Verification items for the finished model (mm, model axes). A direction names the side the tool comes from. Round coordinates to 2 decimals unless told otherwise and drop trailing zeros. Loops run counter-clockwise (first coordinate to the right, second up) from the corner with the lowest first, then second, coordinate; pieces in that order, holes last. Notation, with made-up numbers: M -33,83.25 L -27,83.25 A16 cw -27,99.25 Z; hole C -29,-7 d1. An arc over 180 degrees is marked long. One line per item, written item: value.
Autodesk Inventor part; units mm, degrees
ref_plane "YZ Plane" through (0, 0, 0) normal (1, 0, 0) x (0, 1, 0)
ref_plane "XZ Plane" through (0, 0, 0) normal (0, 1, 0) x (-1, 0, 0)
ref_plane "XY Plane" through (0, 0, 0) normal (0, 0, 1) x (1, 0, 0)
sketch "Sketch1" plane through (0, 0, 0) normal (0, 0, 1) x (1, 0, 0)
  circle A0 centre (0, 0) radius 1.75
  arc A1 (-16.5, -1.75) -> (-16.5, 1.75) centre (-16.5, 0) ccw
  arc A2 (-17.5, 1.75) -> (-17.5, -1.75) centre (-17.5, 0) ccw
  line L0 (-17.5, 1.75) -> (-16.5, 1.75)
  line L1 (-17.5, -1.75) -> (-16.5, -1.75)
  arc A3 (15.9971, -4.4051) -> (14.7172, -7.6627) centre (15.3572, -6.0339) ccw
  arc A4 (15.6479, -8.0283) -> (16.9279, -4.7708) centre (16.2879, -6.3996) ccw
  line L2 (15.6479, -8.0283) -> (14.7172, -7.6627)
  line L3 (16.9279, -4.7708) -> (15.9971, -4.4051)
  circle A5 centre (16.2879, -6.3996) radius 3
  circle A6 centre (-17.5, 0) radius 3
  circle A7 centre (0, 0) radius 2.25
  line L4 (-17.3714, 2.9972) -> (0.0964, 2.2479)
  line L5 (17.2643, -3.5629) -> (0.7323, 2.1275)
  line L6 (-17.6714, -2.9951) -> (-2.0561, -3.8889)
  line L7 (15.3522, -9.2499) -> (0.4916, -4.3714)
  arc A8 (0.4916, -4.3714) -> (-2.0561, -3.8889) centre (-2.6275, -13.8725) ccw
  circle A9 centre (-2.5071, -13.2368) radius 3.25
  circle A10 centre (-2.5071, -13.2368) radius 6
  line L8 (-19.8004, -1.9257) -> (-7.1079, -17.0881)
  line L9 (17.7248, -9.0331) -> (0.3666, -18.5038)
  dimension "d0" = 3.5
  dimension "d1" = 3.5
  dimension "d2" = 3.5
  dimension "d5" = 158.55
  dimension "d7" = 6
  dimension "d9" = 6
  dimension "d10" = 4.5
  dimension "d11" = 10
  dimension "d14" = 0
  dimension "d15" = 0
  dimension "d18" = 6.5
  dimension "d19" = 12
  dimension "d20" = 20
  dimension "d21" = 20
extrude "Extrusion1" add sketch "Sketch1" along normal blind 5
properties part number "CoinLockOpener"
(1) Sectioned sample at C-C on y = 0. Enter the section's corners in (x, z), and give its area (3 significant figures).
Completed:
outline: M -20.5,0 L -19.25,0 L -19.25,5 L -20.5,5 Z; M -14.75,0 L -1.75,0 L -1.75,5 L -14.75,5 Z; M 1.75,0 L 6.91,0 L 6.91,5 L 1.75,5 Z
area: 97.1 mm^2
(2) Sectioned sample at A-A on y = -6. Enter the section's corners in (x, z), and give its area (3 significant figures).
Completed:
outline: M -16.39,0 L 13.61,0 L 13.61,5 L -16.39,5 Z; M 17.99,0 L 19.26,0 L 19.26,5 L 17.99,5 Z
area: 156 mm^2
(3) Sectioned sample at B-B on x = -5. Enter the section's corners in (y, z).
Completed:
outline: M -18.69,0 L -15.32,0 L -15.32,5 L -18.69,5 Z; M -11.15,0 L 2.47,0 L 2.47,5 L -11.15,5 Z
(4) Tool access check on faces 1 (the face through (-8.76, 2.628, 2.465)), 2 (the face through (-17, 1.75, 2)). Record the directions out of +Z, -Z, +X, -X, +Y, -Y that give a thin tool (end or side, any length) a straight path to the whole face; none if there is none.
Completed:
face 1: +Z, -Z, +X, +Y
face 2: +Z, -Z
(5) Mould release check, pull along Y, two halves, no side actions. Record for faces 3 (the face through (-1, -5, 5)), 4 (the face through (9.17, -13.7, 2.46)), 5 (the face through (-17, -1.75, 2)): +Y half, -Y half, draft (parallel to the pull), parting line (faces both ways), or undercut.
Completed:
face 3: draft
face 4: -Y half
face 5: undercut
(6) Thickness scan on L1, parallel to Y at x = 0, z = 3; L2, parallel to X at y = -15, z = 2.5; L3, parallel to Y at x = -4, z = 3.6. Record the ranges inside material, lowest first. Write a range as from..to.
Completed:
L1: y = -18.69..-15.3, -11.17..-1.75, 1.75..2.25
L2: x = -8.86..-5.24, 0.22..6.79
L3: y = -19.05..-16.12, -10.35..2.42
(7) Depth check by flat-ended pin: pin 1 Ø1.5 at (x, z) = (-6.5, 2) entering from +Y; pin 2 Ø0.5 at (x, z) = (-17, 3) entering from -Y; pin 3 Ø2 at (x, z) = (8.5, 2.5) entering from -Y. Enter the tip coordinate at first touch or a pass-through.
Completed:
pin 1: stops at y = 2.56
pin 2: stops at y = -5.57
pin 3: stops at y = -14.61
(8) Sectioned sample at D-D on z = 2.2. Enter the section's corners in (x, y), and give its area (3 significant figures).
Completed:
outline: M -19.8,-1.93 L -7.11,-17.09 A6 ccw 0.37,-18.5 L 17.72,-9.03 A3 ccw 17.26,-3.56 L 0.73,2.13 A2.25 ccw 0.1,2.25 L -17.37,3 A3 ccw Z; hole M -17.5,-1.75 L -16.5,-1.75 A1.75 ccw -16.5,1.75 L -17.5,1.75 A1.75 ccw Z; hole C -2.51,-13.24 d6.5; hole C 0,0 d3.5; hole M 14.72,-7.66 L 15.65,-8.03 A1.75 ccw 16.93,-4.77 L 16,-4.41 A1.75 ccw Z
area: 479 mm^2
